Geometry: final body of the model. Coordinates: model frame, mm. Face numbers are marked on the shaded views. A direction names the side the tool comes from. Coordinates: 2 decimals unless noted, no trailing zeros. Write each loop counter-clockwise with the first axis right and the second up, starting at its lowest first coordinate (ties: lowest second). Pieces come first, ordered by that corner, then holes.
Autodesk Inventor part; units mm, degrees
ref_plane "YZ Plane" through (0, 0, 0) normal (1, 0, 0) x (0, 1, 0)
ref_plane "XZ Plane" through (0, 0, 0) normal (0, 1, 0) x (-1, 0, 0)
ref_plane "XY Plane" through (0, 0, 0) normal (0, 0, 1) x (1, 0, 0)
sketch "Sketch1" plane through (0, 0, 0) normal (0, 0, 1) x (1, 0, 0)
  circle A0 centre (0, 0) radius 3.6
  dimension "d0" = 7.2
extrude "Extrusion1" add sketch "Sketch1" along normal mid plane 83.2
sketch "Sketch2" plane through (0, 0, 41.6) normal (0, 0, 1) x (1, 0, 0)
  circle A0 centre (0, 0) radius 3.6
  line L0 (-3.1177, 1.8) -> (3.1177, 1.8)
  dimension "d3" = 1.8
extrude "Extrusion2" cut sketch "Sketch2" against normal blind 14.4 contours L0 A0 picked at (-0.8728, 2.0235)
sketch "Sketch3" plane through (-3.1177, 1.8, 41.6) normal (0, 1, 0) x (1, 0, 0)
  line L0 (3.1177, 99.84) -> (3.1177, -16.64)
  circle A0 centre (3.1177, 3.2) radius 1.2
  line L1 (6.2354, 0) -> (0, 0)
  point P0 (3.1177, 41.6)
  dimension "d6" = 3.2
  dimension "d7" = 2.4
extrude "Extrusion3" cut sketch "Sketch3" against normal through all
mirror "Mirror1" about plane through (0, 0, 0) normal (0, 0, 1) of "Extrusion2", "Extrusion3"
sketch "Sketch4" plane through (0, 0, 0) normal (1, 0, 0) x (0, 1, 0)
  line L0 (1.8, 27.2) -> (3.6, 27.2)
  line L1 (3.6, -27.2) -> (3.6, 27.2)
  line L2 (1.8, 27.2) -> (3.6, 25.4)
  point P0 (0, 0)
  dimension "d10" = 45
extrude "Extrusion4" cut sketch "Sketch4" along normal through all both and the other way through all
sketch "Sketch5" plane through (0, 0, 41.6) normal (0, 0, 1) x (1, 0, 0)
  line L0 (3.1177, 1.8) -> (-3.1177, 1.8)
  arc A0 (-3.1177, 1.8) -> (3.1177, 1.8) centre (0, 0) ccw
  line L1 (-5.265, 6.8) -> (5.265, 6.8)
  arc A1 (-5.265, 6.8) -> (5.265, 6.8) centre (0, 0) ccw
  dimension "d13" = 5
extrude "Extrusion5" [suppressed]
properties part number "Rear Axle"
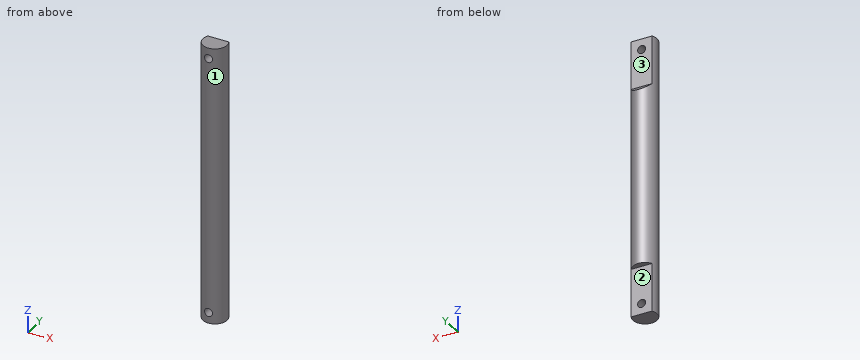
Item 1: Section A-A, the plane x = 0. Output: boundary loops of the cut face in (y, z).
Derived:
outline: (-3.6, -41.6) - (1.8, -41.6) - (1.8, -39.6) - (-3.6, -39.6) - close; (-3.6, -37.2) - (1.8, -37.2) - (1.8, -27.2) - (3.6, -27.2) - (3.6, 25.4) - (1.8, 27.2) - (1.8, 37.2) - (-3.6, 37.2) - close; (-3.6, 39.6) - (1.8, 39.6) - (1.8, 41.6) - (-3.6, 41.6) - close
Item 2: Section B-B, the plane y = 0. Output: boundary loops of the cut face in (x, z).
Derived:
outline: (-3.6, -41.6) - (3.6, -41.6) - (3.6, 41.6) - (-3.6, 41.6) - close; hole circle Ø2.4 at (0, -38.4); hole circle Ø2.4 at (0, 38.4)
Item 3: Section D-D, the plane z = -34. Output: boundary loops of the cut face in (x, y), plus the area to 3 significant figures.
Derived:
outline: (-3.12, 1.8) arc R3.6 ccw (long way) to (3.12, 1.8) - close
area: 32.8 mm2
Item 4: Set-up query: the marked faces 1, 2 and 3. Return all of +Z, -Z, +X, -X, +Y, -Y with unobstructed straight access to the full face (end or side cutting, diameter ignored); none if empty.
Derived:
face 1: +Z, -Z
face 2: -Z, +X, -X, +Y
face 3: +Z, +X, -X, +Y
Item 5: Material intervals for probe 1 along Z at (x, y) = (0, -2.3); probe 2 along X at (y, z) = (0.15, -38.4); probe 3 along X at (y, z) = (-1.25, 38.4), sorted ascending.
Derived:
probe 1: z = -41.6 to -39.6, -37.2 to 37.2, 39.6 to 41.6
probe 2: x = -3.6 to -1.2, 1.2 to 3.6
probe 3: x = -3.38 to -1.2, 1.2 to 3.38
Item 6: Section C-C, the plane z = 38.4. Output: boundary loops of the cut face in (x, y), plus the area to 3 significant figures.
Derived:
outline: (-3.12, 1.8) arc R3.6 ccw to (-1.2, -3.39) - (-1.2, 1.8) - close; (1.2, -3.39) arc R3.6 ccw to (3.12, 1.8) - (1.2, 1.8) - close
area: 20.0 mm2
Item 7: Pin query (flat end, axial travel): pin 1 (3 mm diameter, centred on x = -1.5, z = -38, fed in from +Y); pin 2 (1 mm diameter, centred on y = 1, z = 32, fed in from -X). Return the tip coordinate at first contact, or that it passes through.
Derived:
pin 1: stops at y = 1.8
pin 2: stops at x = -3.57
